The model under review builds one solid part; all positions refer to its coordinate system, in mm. A direction names the side the tool comes from. Give positions to 0.01 mm unless a question says otherwise; leave off trailing zeros. Loops run counter-clockwise (first coordinate to the right, second up) from the corner with the lowest first, then second, coordinate; pieces in that order, holes last. Notation, with made-up numbers: M 56.25,31.5 L 99.25,31.5 A14 ccw 99.25,43.5 Z; hole C 40.25,76.25 d3. An arc over 180 degrees is marked long. One line per item, written item: value. Start each with the question number.
Q1. For pin 1 (11 mm diameter, centred on x = 10.5, z = -10.1, fed in from +Y); pin 2 (17 mm diameter, centred on x = 6.5, z = -13, fed in from -Y); pin 3 (6 mm diameter, centred on x = 12, z = -9, fed in from -Y), all flat-tipped, find the tip position at first contact; note any pin that passes through.
Q2. We need section B-B on y = -21. Write out the cut boundary in (x, z).
Q3. For faces 5 (the face through (15, -50.5, -18)), 6 (the face through (10, -47, 0)), 7 (the face through (6.25, -49, -4)), 8 (the face through (10, -45.5, -16)), 9 (the face through (10, 8.373, -38)), list the 3-axis set-ups (+Z, -Z, +X, -X, +Y, -Y) from which the entire face can be reached by the end or side of a thin tool; tool diameter is ignored.
Q4. To check wall thickness, follow line 1 along X through (y, z) = (2.75, -10.1); line 2 along Y through (x, z) = (8, -5); line 3 along X through (y, z) = (-47, -10). State the ranges of each line that lie inside material, in increasing order. Write a range as from..to.
Q5. We need section C-C on z = -7.5. Write out the cut boundary in (x, y), plus the area to 3 significant figures.
Q6. Mouldability with a two-part tool opening along X and no side actions: class faces 1 (the face through (10, -23, -33)), 2 (the face through (13.64, 3.03, -11.4)), 3 (the face through (16.157, -49.232, -10.057)), 4 (the face through (0, -18, -34)) as released by +X, released by -X, zero draft, split by the parting line, or undercut.
Q7. We need section D-D on x = 18. Write out the cut boundary in (y, z), plus the area to 3 significant figures.
Q8. We need section A-A on x = 10.5. Write out the cut boundary in (y, z).
```python
from build123d import *

# Parameters (mm, degrees)
CYLINDER053_R          = 3.4
CYLINDER053_DEPTH      = 44
CYLINDER052_R          = 5
CYLINDER052_DEPTH      = 9
PAD019_DEPTH           = 5
PAD018_DEPTH           = 21
CUT028_PLACEMENT_ANGLE = 90
SKETCH020_W            = 35
SKETCH020_H            = 62
PAD020_DEPTH           = 3


with BuildPart() as cylinder053:
    # Cylinder053 → Cylinder053 (new body)
    with BuildSketch(Plane(origin=(10.5, -10.1, -9), x_dir=(1, 0, 0), z_dir=(0, 0, 1))):
        Circle(CYLINDER053_R)
    extrude(amount=CYLINDER053_DEPTH)


with BuildPart() as cylinder052:
    # Cylinder052 → Cylinder052 (new body)
    with BuildSketch(Plane(origin=(10.5, -10.1, 44), x_dir=(1, 0, 0), z_dir=(0, 0, 1))):
        Circle(CYLINDER052_R)
    extrude(amount=CYLINDER052_DEPTH)


with BuildPart() as fusion043:
    # Sketch019 → Pad019 (new body)
    with BuildSketch(Plane.XY):
        with BuildLine():
            Line((-4.25, 3.75), (-4.25, 9.25))
            Line((-4.25, 9.25), (-2.65, 17.292388))
            ThreePointArc((2.65, 17.292388), (0, 20), (-2.65, 17.292388))
            Line((2.65, 17.292388), (4.25, 9.25))
            Line((4.25, 3.75), (4.25, 9.25))
            ThreePointArc((4.25, -3.75), (5.657274, 0), (4.25, 3.75))
            Line((4.25, -3.75), (4.25, -9.25))
            Line((2.65, -17.292388), (4.25, -9.25))
            ThreePointArc((-2.65, -17.292388), (0, -20), (2.65, -17.292388))
            Line((-4.25, -9.25), (-2.65, -17.292388))
            Line((-4.25, -3.75), (-4.25, -9.25))
            ThreePointArc((-4.25, 3.75), (-5.657274, 0), (-4.25, -3.75))
        make_face()
    extrude(amount=PAD019_DEPTH)


with BuildPart() as fusion043_1:
    # Body019 placement: moved
    add(fusion043.part.moved(Location((10.5, -10, 48))))

    # Fusion043: union Cylinder052
    add(cylinder052.part)


with BuildPart() as obj1:
    # Sketch018 → Pad018 (new body)
    with BuildSketch(Plane.YZ):
        Polygon((-33, -0.5), (0, -0.5), (0, -5.5), (-38, -5.5), (-38, 50.5), (0, 50.5), (0, 45.5), (-33, 45.5), align=None)
    extrude(amount=PAD018_DEPTH)

    # Cut027: cut Fusion043
    add(fusion043_1.part, mode=Mode.SUBTRACT)

    # Cut028: cut Cylinder053
    add(cylinder053.part, mode=Mode.SUBTRACT)


with BuildPart() as obj1_1:
    # Cut028 placement: moved
    add(obj1.part.rotate(Axis((0, 0, 0), (1, 0, 0)), CUT028_PLACEMENT_ANGLE))


with BuildPart() as fusion044:
    # Sketch020 → Pad020 (new body)
    with BuildSketch(Plane.XY):
        with Locations((10.548899, -22.627238)):
            Rectangle(SKETCH020_W, SKETCH020_H)
    extrude(amount=PAD020_DEPTH)


with BuildPart() as fusion044_1:
    # Body020 placement: moved
    add(fusion044.part.moved(Location((0, 0, -39))))

    # Fusion044: union obj1
    add(obj1_1.part)


solid = fusion044_1.part
```
Solved:
1. pin 1: y = 5.5
1. pin 2: y = -50.5
1. pin 3: y = 0.5
2. outline: M -6.95,-39 L 28.05,-39 L 28.05,-36 L 21,-36 L 21,-33 L 0,-33 L 0,-36 L -6.95,-36 Z
3. face 5: +Z, +X, -X, -Y
3. face 6: +Z, +X, -X, +Y, -Y
3. face 7: -Y
3. face 8: +Z, +X, -X
3. face 9: +Z, -Z, +X, -X, +Y
4. line 1: 0..7.1, 13.9..21
4. line 2: -48..-45.5, 0.5..5.5
4. line 3: 0..5.5, 15.5..21
5. outline: M 0,-50.5 L 5.42,-50.5 L 5.42,-48 L 6.23,-48 L 6.23,-45.5 L 0,-45.5 Z; M 0,0.5 L 8.31,0.5 L 8.31,5.5 L 0,5.5 Z; M 12.69,0.5 L 21,0.5 L 21,5.5 L 12.69,5.5 Z; M 14.77,-48 L 15.58,-48 L 15.58,-50.5 L 21,-50.5 L 21,-45.5 L 14.77,-45.5 Z
5. area: 141 mm2
6. face 1: zero draft
6. face 2: undercut
6. face 3: undercut
6. face 4: released by -X
7. outline: M -53.63,-39 L 8.37,-39 L 8.37,-36 L 5.5,-36 L 5.5,0 L 0.5,0 L 0.5,-33 L -45.5,-33 L -45.5,0 L -50.5,0 L -50.5,-36 L -53.63,-36 Z
7. area: 684 mm2
8. outline: M -53.63,-39 L 8.37,-39 L 8.37,-36 L 5.5,-36 L 5.5,-13.5 L 0.5,-13.5 L 0.5,-33 L -45.5,-33 L -45.5,-15.1 L -48,-15.1 L -48,-30 L -50.5,-30 L -50.5,-36 L -53.63,-36 Z; M -48,-5.1 L -45.5,-5.1 L -45.5,0 L -48,0 Z; M 0.5,-6.7 L 5.5,-6.7 L 5.5,0 L 0.5,0 Z
